Autodesk Inventor part; units mm, degrees
ref_plane "Work Plane1" through (0, 0, -15) normal (0, 0, 1) x (1, 0, 0)
ref_plane "YZ Plane" through (0, 0, 0) normal (1, 0, 0) x (0, 1, 0)
ref_plane "XZ Plane" through (0, 0, 0) normal (0, 1, 0) x (-1, 0, 0)
sketch "Sketch1" plane through (0, 0, 0) normal (0, 0, 1) x (1, 0, 0)
  line L0 (0, 0) -> (25, 0)
  line L1 (25, 0) -> (25, 40)
  line L2 (25, 40) -> (0, 40)
  line L3 (0, 40) -> (0, 0)
  dimension "d1" = 25
  dimension "d2" = 40
  dimension "d3" = 25
extrude "Extrusion1" add sketch "Sketch1" against normal blind 30
sketch "Sketch2" plane through (25, 0, 0) normal (1, 0, 0) x (0, 0, -1)
  line L0 (0, 0) -> (30, 0)
  circle A0 centre (15, 6.56) radius 2.46
extrude "Extrusion2" cut sketch "Sketch2" against normal blind 30
sketch "Sketch3" plane through (0, 0, 0) normal (-1, 0, 0) x (0, 0, 1)
  line L0 (0, 0) -> (-30, 0)
  line L1 (-25.05, 0) -> (-4.95, 0)
  line L2 (-4.95, 0) -> (-4.95, 33.12)
  line L3 (-4.95, 33.12) -> (-25.05, 33.12)
  line L4 (-25.05, 33.12) -> (-25.05, 0)
  dimension "d11" = 20.1
extrude "Extrusion3" cut sketch "Sketch3" against normal blind 20
sketch "Sketch4" plane through (0, 0, 0) normal (0, -1, 0) x (1, 0, 0)
  line L0 (20, -4.95) -> (20, -25.05)
  line L1 (20, -15) -> (25, -15)
  line L2 (25, 0) -> (25, -30)
  line L3 (20, -8.025) -> (25, -8.025)
  line L4 (25, -8.025) -> (25, -21.975)
  line L5 (25, -21.975) -> (20, -21.975)
  line L6 (20, -21.975) -> (20, -8.025)
  line L7 (20, -8.025) -> (25, -21.975) construction
  line L8 (25, -8.025) -> (20, -21.975) construction
  line L9 (25, -12.54) -> (25, -17.46)
  point P0 (0, 0)
  point P1 (22.5, -15)
  dimension "d14" = 13.95
extrude "Extrusion4" add sketch "Sketch4" along normal blind 15
sketch "Sketch5" plane through (20, 0, 0) normal (-1, 0, 0) x (0, 0, 1)
  circle A0 centre (-15, 6.56) radius 2.46
  circle A1 centre (-15, 6.56) radius 4.7025
  circle A2 centre (-15, 6.56) radius 2.46
  circle A3 centre (-15, 6.56) radius 2.46
  point P0 (0, 0)
  dimension "d17" = 9.405
extrude "Extrusion5" cut sketch "Sketch5" against normal blind 2.1
sketch "Sketch6" plane through (25, 0, 0) normal (1, 0, 0) x (0, 0, -1)
  circle A0 centre (15, 6.56) radius 4.7025
  line L0 (15, 6.56) -> (15, 23.56)
  circle A1 centre (15, 23.56) radius 2.46
  point P0 (0, 0)
  dimension "d20" = 17
  dimension "d21" = 4.92
extrude "Extrusion6" cut sketch "Sketch6" against normal blind 10 contours A1
sketch "Sketch7" plane through (20, 0, 0) normal (-1, 0, 0) x (0, 0, 1)
  circle A0 centre (-15, 23.56) radius 2.46
  circle A1 centre (-15, 23.56) radius 4.7025
  point P0 (0, 0)
  dimension "d24" = 9.405
extrude "Extrusion7" cut sketch "Sketch7" against normal blind 2.1
sketch "Sketch9" plane through (25, 0, 0) normal (1, 0, 0) x (0, 0, -1)
  circle A0 centre (15, 6.56) radius 2.46
  circle A1 centre (15, 6.56) radius 2.46
  circle A2 centre (15, 23.56) radius 2.46
  circle A3 centre (15, 23.56) radius 2.46
  line L0 (30, 40) -> (30, 0)
  line L1 (30, 0) -> (30, 40)
  line L2 (30, 40) -> (0, 40)
  line L3 (0, 40) -> (0, 0)
  line L4 (0, 0) -> (8.025, 0)
  line L5 (21.975, 0) -> (21.975, -15)
  line L6 (21.975, -15) -> (8.025, -15)
  line L7 (8.025, -15) -> (8.025, 0)
  line L8 (0, 0) -> (8.025, 0)
  line L9 (21.975, 0) -> (30, 0)
extrude "Extrusion8" add sketch "Sketch9" along normal blind 5
sketch "Sketch10" plane through (0, 40, 0) normal (0, 1, 0) x (1, 0, 0)
  line L0 (0, 30) -> (30, 30)
  line L1 (30, 0) -> (0, 0)
  line L2 (0, 30) -> (30, 30)
  line L3 (30, 30) -> (30, 0)
  line L4 (30, 0) -> (0, 0)
  line L5 (0, 0) -> (0, 30)
extrude "Extrusion9" add sketch "Sketch10" along normal blind 30
sketch "Sketch12" plane through (30, 0, 0) normal (1, 0, 0) x (0, 0, -1)
  circle A0 centre (15, 6.56) radius 2.46
  line L0 (15, 6.56) -> (15, 15.06)
  circle A1 centre (15, 15.06) radius 2.525
  point P0 (0, 0)
  dimension "d31" = 8.5
  dimension "d33" = 5.05
extrude "Extrusion10" cut sketch "Sketch12" against normal blind 30 contours A1
sketch "Sketch14" plane through (0, 0, 0) normal (0, 0, 1) x (1, 0, 0)
  line L0 (30, 70) -> (0, 70)
  line L1 (0, 70) -> (0, 85)
  line L2 (-15, 100) -> (-23, 100)
  line L3 (30, 0) -> (30, 70)
  line L4 (30, 100) -> (30, 70)
  arc A0 (0, 85) -> (-15, 100) centre (-15, 85) ccw
  line L5 (-23, 120) -> (15, 120)
  line L6 (-20.5, 118) -> (-18, 110)
  line L7 (-20.5, 118) -> (-23, 120)
  line L8 (-20.5, 102) -> (-18, 110)
  line L9 (-20.5, 102) -> (-23, 100)
  line L10 (30, 105) -> (15, 120)
  line L11 (30, 105) -> (30, 100)
  point P0 (0, 0)
  point P1 (0, 100)
  dimension "d47" = 30
  dimension "d54" = 15
  dimension "d60" = 20
extrude "Extrusion12" add sketch "Sketch14" against normal blind 30
sketch "Sketch15" plane through (0, 0, -25.05) normal (-1, 0, 0) x (0, 0, 1)
  line L0 (0, 33.12) -> (20.1, 33.12)
  line L1 (20.1, 33.12) -> (20.1, 0)
  line L2 (0, 33.12) -> (20.1, 33.12)
  line L3 (20.1, 33.12) -> (20.1, 31.1)
  line L4 (20.1, 31.1) -> (0, 31.1)
  line L5 (0, 31.1) -> (0, 33.12)
  point P0 (25.05, 0)
  dimension "d57" = 2.02
extrude "Extrusion13" add sketch "Sketch15" against normal blind 20
sketch "Sketch19" plane through (0, 0, 0) normal (0, 0, 1) x (1, 0, 0)
  arc A0 (0, 85) -> (-15, 100) centre (-15, 85) ccw
  arc A1 (0, 85) -> (-15, 100) centre (-15, 85) ccw
  line L0 (-15, 100) -> (-23, 100)
  line L1 (-15, 100) -> (-23, 100)
  line L2 (-23, 100) -> (-20.5, 102)
  line L3 (-23, 100) -> (-20.5, 102)
  line L4 (-20.5, 102) -> (-18, 110)
  line L5 (-20.5, 102) -> (-18, 110)
  line L6 (-18, 110) -> (-20.5, 118)
  line L7 (-18, 110) -> (-20.5, 118)
  line L8 (-23, 120) -> (15, 120)
  line L9 (-20.5, 118) -> (-23, 120)
  line L10 (-23, 120) -> (15, 120)
  line L11 (15, 120) -> (30, 105)
  line L12 (15, 120) -> (30, 105)
  line L13 (30, 105) -> (30, 85)
  line L14 (30, 0) -> (30, 105)
  line L15 (0, 85) -> (30, 85)
  point P0 (0, 0)
extrude "Extrusion14" add sketch "Sketch19" along normal blind 45
ref_plane "Work Plane1" through (0, 0, -15) normal (0, 0, 1) x (1, 0, 0)
mirror "Mirror1" about plane through (0, 0, -15) normal (0, 0, 1) of "Extrusion14"
properties part number "16mm_x_120mm"
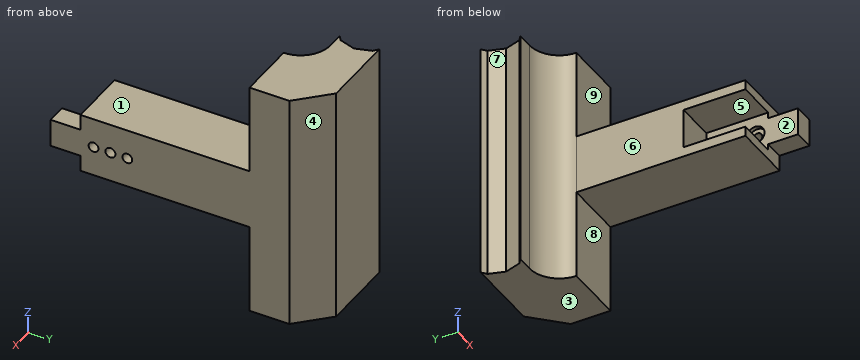
Here's how the part is built. I have some questions about the finished solid (model axes, mm). Face numbers are marked on the shaded views. A direction names the side the tool comes from. Coordinates: 2 decimals unless noted, no trailing zeros. Loops run counter-clockwise (first coordinate to the right, second up) from the corner with the lowest first, then second, coordinate; pieces in that order, holes last.
1. I need wall thicknesses on L1, parallel to Y at x = 25, z = -15 (3 decimals); L2, parallel to Y at x = 26.75, z = -15 (3 decimals); L3, parallel to Z at x = 21, y = 6. Which ranges of each line are inside material? Lowest first, please.
2. Imagine slicing it at D-D, the plane z = 24. Please give me the cut outline in (x, y).
3. Imagine slicing it at C-C, the plane x = 17. Please give me the cut outline in (y, z), and give its area (3 significant figures).
4. Imagine slicing it at A-A, the plane z = -15. Count the separate pieces of the cut face and the enclosed holes in it, and give its area (3 significant figures).
5. For P1, Ø8, axis at x = 24.5, y = -8.5, coming from the -Z side (3 decimals); P2, Ø8, axis at x = -1.5, y = 80, coming from the -Z side; P3, Ø2.5, axis at x = 14, z = -27, coming from the -Y side, each with a flat end and sliding along its axis, tell me the tip position at first contact or that it passes through.
6. If we mould it in two halves opening along Z, with no side actions, what happens to the marked faces 1, 2, 3 and 4? For each: pulls with the +Z half, pulls with the -Z half, needs draft (parallel to the pull), parting line crosses it, or undercut.
7. For the marked faces 5, 6, 7, 8 and 9, which set-ups out of +Z, -Z, +X, -X, +Y, -Y let a thin tool reach every point of the face, with its end or its side?
8. Imagine slicing it at B-B, the plane y = 15.06. Please give me the cut outline in (x, z) (3 decimals).
Taken from the geometry:
1. L1: y = -15 to 4.1, 9.02 to 12.535, 17.585 to 21.1, 26.02 to 110
1. L2: y = -15 to 4.1, 9.02 to 12.535, 17.585 to 21.1, 26.02 to 108.25
1. L3: z = -30 to -19.67, -10.33 to 0
2. outline: (-23, 100) - (-15, 100) arc R15 cw to (0, 85) - (30, 85) - (30, 105) - (15, 120) - (-23, 120) - (-20.5, 118) - (-18, 110) - (-20.5, 102) - close
3. outline: (0, -30) - (85, -30) - (85, -75) - (118, -75) - (118, 45) - (85, 45) - (85, 0) - (0, 0) - (0, -4.95) - (31.1, -4.95) - (31.1, -25.05) - (0, -25.05) - close
3. area: 5,880 mm2
4. separate pieces: 4
4. enclosed holes: 0
4. area: 3,290 mm2
5. P1: stops at z = -21.975
5. P2: stops at z = -30
5. P3: stops at y = 0
6. face 1: pulls with the +Z half
6. face 2: undercut
6. face 3: pulls with the -Z half
6. face 4: needs draft
7. face 5: -X, -Y
7. face 6: +Z, -Z, -X, -Y
7. face 7: +Z, -Z, -X
7. face 8: -Z, +X, -X, -Y
7. face 9: +Z, +X, -X, -Y
8. outline: (0, -30) - (30, -30) - (30, -17.525) - (20, -17.525) - (20, -25.05) - (0, -25.05) - close; (0, -4.95) - (20, -4.95) - (20, -12.475) - (30, -12.475) - (30, 0) - (0, 0) - close
